The model under review builds one solid part; all positions refer to its coordinate system, in mm. A direction names the side the tool comes from. Give positions to 0.01 mm unless a question says otherwise; leave off trailing zeros. Order: outer loops, then holes, each group sorted by start corner. A loop starts at its lowest first (then second) coordinate and runs counter-clockwise, first axis right, second up. Notation, with made-up numbers: (74.25, 76.5) -> (82.25, 76.5) arc R10 cw to (82.25, 82.5) -> close; hole circle Ø9 at (36, 21). An arc over 180 degrees is marked (long way). Use one line per item in the form item = value.
```python
from build123d import *

# Parameters (mm, degrees)
F1_DEPTH = 10
F2_W     = 8
F2_H     = 8
F3_DEPTH = 150
F4_R     = 1
F5_DEPTH = 25
F6_W     = 2
F6_H     = 10
F7_DEPTH = 25


with BuildPart() as f1:
    # F0 (on Top) → F1 (new body)
    with BuildSketch(Plane.XY):
        Polygon((8.409432, 76.851626), (-1.590568, 76.851626), (-1.590568, -33.148374), (8.409432, -53.148374), align=None)
    extrude(amount=F1_DEPTH)

    # F2 (on face) → F3 (cut)
    with BuildSketch(Plane(origin=(0, 76.851626, 0), x_dir=(-1, 0, 0), z_dir=(0, 1, 0))):
        with Locations((-3.409432, 5)):
            Rectangle(F2_W, F2_H)
    extrude(amount=-F3_DEPTH, mode=Mode.SUBTRACT)

    # F4 (on face) → F5 (cut)
    with BuildSketch(Plane.XY.offset(10)):
        with BuildLine():
            ThreePointArc((-1.590568, 71.851626), (3.409432, 76.851626), (8.409432, 71.851626))
            Line((8.409432, 71.851626), (14.622306, 71.851626))
            Line((14.622306, 71.851626), (14.622306, 78.704596))
            Line((14.622306, 78.704596), (-2.961113, 78.068092))
            Line((-2.961113, 78.068092), (-2.736083, 71.851626))
            Line((-2.736083, 71.851626), (-1.590568, 71.851626))
        make_face()
        with Locations((3.409432, 71.851626)):
            Circle(F4_R)
    extrude(amount=-F5_DEPTH, mode=Mode.SUBTRACT)

    # F6 (on face) → F7 (cut)
    with BuildSketch(Plane.YZ.offset(8.409432)):
        Polygon((-51.148374, 19.7851), (-54.233824, 19.7851), (-54.233824, -10.105174), (-51.148374, -10.105174), (-51.148374, 0), (-53.148374, 0), (-53.148374, 10), (-51.148374, 10), align=None)
        with Locations((-52.148374, 5)):
            Rectangle(F6_W, F6_H)
    extrude(amount=-F7_DEPTH, mode=Mode.SUBTRACT)


solid = f1.part
```
1. Add section C-C on x = 0.5. Give the boundary of the cut face in (y, z), then the cut area to 3 significant figures.
Values:
outline = (-37.33, 0) -> (75.92, 0) -> (75.92, 1) -> (-37.33, 1) -> close; (-37.33, 9) -> (75.92, 9) -> (75.92, 10) -> (-37.33, 10) -> close
area = 226 mm^2
2. Tool access review of faces 1 (the face through (3, 14, 9)), 2 (the face through (-1.591, 20, 5)): name each direction out of +Z, -Z, +X, -X, +Y, -Y from which nothing blocks a thin tool from reaching the whole face with its end or side.
Values:
face_1 = +Y, -Y
face_2 = +Z, -Z, -X, +Y, -Y
3. Add section B-B on y = -10.5. Give the boundary of the cut face in (x, z), then the cut area to 3 significant figures.
Values:
outline = (-1.59, 0) -> (8.41, 0) -> (8.41, 10) -> (-1.59, 10) -> close; hole (-0.59, 1) -> (7.41, 1) -> (7.41, 9) -> (-0.59, 9) -> close
area = 36.0 mm^2
4. Add section A-A on z = 5.25. Give the boundary of the cut face in (x, y).
Values:
outline = (-1.59, -33.15) -> (-0.59, -35.15) -> (-0.59, 74.85) arc R5 ccw to (-1.59, 71.85) -> close; (7.41, -51.15) -> (8.41, -51.15) -> (8.41, 71.85) arc R5 ccw to (7.41, 74.85) -> close
5. The part is to be moulded in two halves that separate along X. For faces 3 (the face through (8.409, 9, 5)), 4 (the face through (7.409, 13, 5)), 5 (the face through (-0.975, 74.256, 5.07)), say which applies: +X half, -X half, draft (parallel to the pull), parting line (faces both ways), or undercut.
Values:
face_3 = +X half
face_4 = undercut
face_5 = parting line
6. For L1, parallel to Z at x = 6.75, y = 62.5; L2, parallel to X at y = 24, z = 5.75; L3, parallel to X at y = -43, z = 3, list the stretches that pass through material, from the lowest coordinate up.
Values:
L1 = 0 to 1, 9 to 10
L2 = -1.59 to -0.59, 7.41 to 8.41
L3 = 7.41 to 8.41
7. For pin 1 Ø1.5 at (y, z) = (-34.5, 1.5) entering from -X; pin 2 Ø3 at (x, z) = (0.5, 4) entering from -Y, all flat-tipped, find the tip position at first contact; note any pin that passes through.
Values:
pin_1 = -1.29
pin_2 = -35.15
